```python
from build123d import *

# Parameters (mm, degrees)
SKETCH1_W           = 12.9
SKETCH1_H           = 3.3782
BOSS_EXTRUDE2_DEPTH = 3.175


with BuildPart() as part:
    # Sketch1 → Boss-Extrude2 (new body)
    with BuildSketch(Plane.XY):
        Polygon((6.2500002, -9.525), (6.2500002, -3.2782), (406.4, -3.2782), (406.4, 126.6968), (6.2500002, 126.6968), (6.2500002, 132.9436), (0, 132.9436), (0, -9.525), align=None)
        with Locations((19.05, 121.8327)):
            Rectangle(SKETCH1_W, SKETCH1_H, mode=Mode.SUBTRACT)
        with Locations((45.357142857, 121.8327)):
            Rectangle(SKETCH1_W, SKETCH1_H, mode=Mode.SUBTRACT)
        with Locations((387.35, 121.8327)):
            Rectangle(SKETCH1_W, SKETCH1_H, mode=Mode.SUBTRACT)
        with Locations((361.042857143, 121.8327)):
            Rectangle(SKETCH1_W, SKETCH1_H, mode=Mode.SUBTRACT)
        with Locations((71.664285714, 121.8327)):
            Rectangle(SKETCH1_W, SKETCH1_H, mode=Mode.SUBTRACT)
        with Locations((97.971428571, 121.8327)):
            Rectangle(SKETCH1_W, SKETCH1_H, mode=Mode.SUBTRACT)
        with Locations((124.278571429, 121.8327)):
            Rectangle(SKETCH1_W, SKETCH1_H, mode=Mode.SUBTRACT)
        with Locations((150.585714286, 121.8327)):
            Rectangle(SKETCH1_W, SKETCH1_H, mode=Mode.SUBTRACT)
        with Locations((176.892857143, 121.8327)):
            Rectangle(SKETCH1_W, SKETCH1_H, mode=Mode.SUBTRACT)
        with Locations((203.2, 121.8327)):
            Rectangle(SKETCH1_W, SKETCH1_H, mode=Mode.SUBTRACT)
        with Locations((229.507142857, 121.8327)):
            Rectangle(SKETCH1_W, SKETCH1_H, mode=Mode.SUBTRACT)
        with Locations((255.814285714, 121.8327)):
            Rectangle(SKETCH1_W, SKETCH1_H, mode=Mode.SUBTRACT)
        with Locations((282.121428571, 121.8327)):
            Rectangle(SKETCH1_W, SKETCH1_H, mode=Mode.SUBTRACT)
        with Locations((308.428571429, 121.8327)):
            Rectangle(SKETCH1_W, SKETCH1_H, mode=Mode.SUBTRACT)
        with Locations((334.735714286, 121.8327)):
            Rectangle(SKETCH1_W, SKETCH1_H, mode=Mode.SUBTRACT)
        with Locations((387.35, 1.5859)):
            Rectangle(SKETCH1_W, SKETCH1_H, mode=Mode.SUBTRACT)
        with Locations((361.042857143, 1.5859)):
            Rectangle(SKETCH1_W, SKETCH1_H, mode=Mode.SUBTRACT)
        with Locations((334.735714286, 1.5859)):
            Rectangle(SKETCH1_W, SKETCH1_H, mode=Mode.SUBTRACT)
        with Locations((308.428571429, 1.5859)):
            Rectangle(SKETCH1_W, SKETCH1_H, mode=Mode.SUBTRACT)
        with Locations((282.121428571, 1.5859)):
            Rectangle(SKETCH1_W, SKETCH1_H, mode=Mode.SUBTRACT)
        with Locations((255.814285714, 1.5859)):
            Rectangle(SKETCH1_W, SKETCH1_H, mode=Mode.SUBTRACT)
        with Locations((229.507142857, 1.5859)):
            Rectangle(SKETCH1_W, SKETCH1_H, mode=Mode.SUBTRACT)
        with Locations((203.2, 1.5859)):
            Rectangle(SKETCH1_W, SKETCH1_H, mode=Mode.SUBTRACT)
        with Locations((176.892857143, 1.5859)):
            Rectangle(SKETCH1_W, SKETCH1_H, mode=Mode.SUBTRACT)
        with Locations((150.585714286, 1.5859)):
            Rectangle(SKETCH1_W, SKETCH1_H, mode=Mode.SUBTRACT)
        with Locations((124.278571429, 1.5859)):
            Rectangle(SKETCH1_W, SKETCH1_H, mode=Mode.SUBTRACT)
        with Locations((97.971428571, 1.5859)):
            Rectangle(SKETCH1_W, SKETCH1_H, mode=Mode.SUBTRACT)
        with Locations((71.664285714, 1.5859)):
            Rectangle(SKETCH1_W, SKETCH1_H, mode=Mode.SUBTRACT)
        with Locations((45.357142857, 1.5859)):
            Rectangle(SKETCH1_W, SKETCH1_H, mode=Mode.SUBTRACT)
        with Locations((19.05, 1.5859)):
            Rectangle(SKETCH1_W, SKETCH1_H, mode=Mode.SUBTRACT)
    extrude(amount=BOSS_EXTRUDE2_DEPTH)


solid = part.part
```
The model under review builds one solid part; all positions refer to its coordinate system, in mm. Coordinates: 2 decimals unless noted, no trailing zeros. Order: outer loops, then holes, each group sorted by start corner. A loop starts at its lowest first (then second) coordinate and runs counter-clockwise, first axis right, second up. Notation, with made-up numbers: (25.5, -24) -> (39.5, -24) arc R16 ccw to (39.5, 7) -> close; hole circle Ø4 at (-33, 7.5). An arc over 180 degrees is marked (long way). Answer in a Markdown table with one row per item. Add a question column.
Item 1: Clearance check with flat-ended pins moving along their axes: pin 1 (1.6 mm diameter, centred on x = 18, z = 2, fed in from +Y); pin 2 (1.5 mm diameter, centred on x = 181.5, z = 1.5, fed in from -Y). State where each tip first meets the part, or that it passes through.
Item 2: To check wall thickness, follow probe 1 along Y at (x, z) = (74.5, 1.95) (3 decimals); probe 2 along Y at (x, z) = (193, 0.4). State the ranges of each line that lie inside material, in increasing order.
Item 3: We need section B-B on x = 86. Write out the cut boundary in (y, z) (3 decimals).
Item 4: We need section A-A on z = 1.6. Give the number of separate pieces and of enclosed holes in the cut face, plus the area to 3 significant figures.
Final values:
| question | item | result |
|---|---|---|
| 1 | pin 1 | stops at y = 126.7 |
| 1 | pin 2 | stops at y = -3.28 |
| 2 | probe 1 | y = -3.278 to -0.103, 3.275 to 120.144, 123.522 to 126.697 |
| 2 | probe 2 | y = -3.28 to 126.7 |
| 3 | outline | (-3.278, 0) -> (126.697, 0) -> (126.697, 3.175) -> (-3.278, 3.175) -> close |
| 4 | separate pieces | 1 |
| 4 | enclosed holes | 30 |
| 4 | area | 51,600 mm2 |
